```python
from build123d import *

# Parameters (mm, degrees)
F0_W     = 1220
F0_H     = 515
F1_DEPTH = 20
F2_W     = 1200
F2_H     = 8
F3_DEPTH = 30
F4_W     = 8
F4_H     = 492
F5_DEPTH = 30
F6_W     = 8
F6_H     = 492
F7_DEPTH = 30


with BuildPart() as f1:
    # F0 (on Top) → F1 (new body, symmetric)
    with BuildSketch(Plane.XY):
        Rectangle(F0_W, F0_H)
    extrude(amount=F1_DEPTH, both=True)

    # F2 (on face) → F3 (cut)
    with BuildSketch(Plane.XY.offset(20)):
        with Locations((0, 243.5)):
            Rectangle(F2_W, F2_H)
    extrude(amount=-F3_DEPTH, mode=Mode.SUBTRACT)

    # F4 (on face) → F5 (cut)
    with BuildSketch(Plane.XY.offset(20)):
        with Locations((-596, -6.5)):
            Rectangle(F4_W, F4_H)
    extrude(amount=-F5_DEPTH, mode=Mode.SUBTRACT)

    # F6 (on face) → F7 (cut)
    with BuildSketch(Plane.XY.offset(20)):
        with Locations((596, -6.5)):
            Rectangle(F6_W, F6_H)
    extrude(amount=-F7_DEPTH, mode=Mode.SUBTRACT)


solid = f1.part
```
Geometry: final body of the model. Coordinates: model frame, mm. A direction names the side the tool comes from. Coordinates: 2 decimals unless noted, no trailing zeros. Order: outer loops, then holes, each group sorted by start corner. A loop starts at its lowest first (then second) coordinate and runs counter-clockwise, first axis right, second up. Notation, with made-up numbers: M -9,37 L 45,37 A17 cw 45,58 Z; hole C 9.5,53.25 d7. An arc over 180 degrees is marked long. Answer in a Markdown table with one row per item. Add a question column.
Q1. Section query A-A on z = -1. Return the cut outline in (x, y), and give its area (3 significant figures).
Q2. Mould query, pull axis X, two halves, no side actions, for faces 1 (the flat face through (610, -4, 0)), 2 (the flat face through (-8, 247.5, 5)), 3 (the flat face through (-9, -257.5, 0)). Classes: released by +X, released by -X, zero draft, split by the parting line, or undercut.
Q3. Reachability of faces 4 (the flat face through (-9, 4, 20)), 5 (the flat face through (-600, -6, 5)) from +Z, -Z, +X, -X, +Y, -Y: full face, straight path, thin tool, end or side. Return the list, or none.
Q4. Line query: L1, parallel to X at y = 230, z = 5.5; L2, parallel to Y at x = -515.5, z = -1.5. Output: solid intervals per line, ascending.
Completed:
| question | item | result |
|---|---|---|
| 1 | outline | M -610,-257.5 L 610,-257.5 L 610,257.5 L -610,257.5 Z; hole M -600,-252.5 L -592,-252.5 L -592,239.5 L 592,239.5 L 592,-252.5 L 600,-252.5 L 600,247.5 L -600,247.5 Z |
| 1 | area | 611,000 mm2 |
| 2 | face 1 | released by +X |
| 2 | face 2 | undercut |
| 2 | face 3 | zero draft |
| 3 | face 4 | +Z, +X, -X, +Y, -Y |
| 3 | face 5 | +Z |
| 4 | L1 | x = -610 to -600, -592 to 592, 600 to 610 |
| 4 | L2 | y = -257.5 to 239.5, 247.5 to 257.5 |
